Check sheet for the modelled part. Datum: model origin and axes. Units: mm. Round coordinates to 2 decimals unless told otherwise and drop trailing zeros. Order: outer loops, then holes, each group sorted by start corner. A loop starts at its lowest first (then second) coordinate and runs counter-clockwise, first axis right, second up. Notation, with made-up numbers: (-8, -1.5) -> (4, -1.5) arc R13 ccw to (4, 22.5) -> close; hole circle Ø8 at (-38.75, 19.5). An arc over 180 degrees is marked (long way). Answer in a Markdown table with one row per item. Add a question column.
1. Sectioned sample at D-D, the plane z = -24. Record the boundary of the cut face in (x, y), then the cut area to 3 significant figures.
2. Sectioned sample at B-B, the plane x = -32. Record the boundary of the cut face in (y, z).
3. Depth check by flat-ended pin: P1, Ø1.8, axis at x = 34.34, z = -80.5, coming from the +Y side. Enter the tip coordinate at first touch or a pass-through.
4. Sectioned sample at C-C, the plane x = 23. Record the boundary of the cut face in (y, z).
5. Sectioned sample at A-A, the plane z = -131. Record the boundary of the cut face in (x, y).
6. Material ranges on L1, parallel to X at y = 1.05, z = -55.5; L2, parallel to Z at x = -9.5, y = 0.45; L3, parallel to X at y = 1.65, z = -84, recorded low to high. Write a range as from..to.
Autodesk Inventor part; units mm, degrees
ref_plane "YZ Plane" through (0, 0, 0) normal (1, 0, 0) x (0, 1, 0)
ref_plane "XZ Plane" through (0, 0, 0) normal (0, 1, 0) x (-1, 0, 0)
ref_plane "XY Plane" through (0, 0, 0) normal (0, 0, 1) x (1, 0, 0)
sketch "Sketch1" plane through (0, 0, 0) normal (0, 1, 0) x (-1, 0, 0)
  line L0 (37.7589, 9.4959) -> (-42.2411, 9.4959)
  line L1 (-42.2411, 9.4959) -> (-42.2411, -290.5041)
  line L2 (-42.2411, -290.5041) -> (37.7589, -290.5041)
  line L3 (27.7589, -20.5041) -> (1.7589, -20.5041)
  line L4 (1.7589, -20.5041) -> (1.7589, -65.5041)
  line L5 (1.7589, -65.5041) -> (27.7589, -65.5041)
  line L6 (27.7589, -65.5041) -> (27.7589, -20.5041)
  line L7 (-8.2411, -20.5041) -> (-34.2411, -20.5041)
  line L8 (-34.2411, -20.5041) -> (-34.2411, -65.5041)
  line L9 (-34.2411, -65.5041) -> (-8.2411, -65.5041)
  line L10 (-8.2411, -65.5041) -> (-8.2411, -20.5041)
  line L11 (-6.2411, -81.8041) -> (-32.2411, -81.8041)
  line L12 (-32.2411, -81.8041) -> (-32.2411, -156.8041)
  line L13 (-32.2411, -156.8041) -> (-6.2411, -156.8041)
  line L14 (-6.2411, -156.8041) -> (-6.2411, -81.8041)
  circle A0 centre (-3.3411, -80.5041) radius 1.5
  circle A1 centre (-34.3411, -80.5041) radius 1.5
  circle A2 centre (-3.3411, -155.5041) radius 1.5
  circle A3 centre (-34.3411, -155.5041) radius 1.5
  line L15 (37.7589, 9.4959) -> (37.7589, -110.5041)
  line L16 (37.7589, -110.5041) -> (7.7589, -110.5041)
  line L17 (7.7589, -110.5041) -> (7.7589, -170.5041)
  line L18 (7.7589, -170.5041) -> (37.7589, -170.5041)
  line L19 (37.7589, -170.5041) -> (37.7589, -290.5041)
  line L20 (12.7589, -238.5041) -> (-17.2411, -238.5041)
  line L21 (-17.2411, -238.5041) -> (-17.2411, -260.5041)
  line L22 (-17.2411, -260.5041) -> (12.7589, -260.5041)
  line L23 (12.7589, -260.5041) -> (12.7589, -238.5041)
  line L24 (12.7589, -210.5041) -> (-6.2411, -210.5041)
  line L25 (-6.2411, -210.5041) -> (-6.2411, -223.5041)
  line L26 (-6.2411, -223.5041) -> (12.7589, -223.5041)
  line L27 (12.7589, -223.5041) -> (12.7589, -210.5041)
  circle A4 centre (-7.2411, -275.5041) radius 1.5
  circle A5 centre (-7.2411, -5.5041) radius 1.5
  point P0 (0, 0)
  dimension "d0" = 300
  dimension "d1" = 80
  dimension "d4" = 45
  dimension "d5" = 26
  dimension "d6" = 30
  dimension "d8" = 45
  dimension "d9" = 26
  dimension "d10" = 30
  dimension "d11" = 10
  dimension "d12" = 75
  dimension "d13" = 26
  dimension "d16" = 1.3
  dimension "d17" = 2.9
  dimension "d18" = 3
  dimension "d20" = 31
  dimension "d22" = 3
  dimension "d23" = 75
  dimension "d24" = 3
  dimension "d25" = 75
  dimension "d26" = 3
  dimension "d27" = 15
  dimension "d28" = 10
  dimension "d29" = 120
  dimension "d30" = 120
  dimension "d31" = 30
  dimension "d32" = 22
  dimension "d33" = 30
  dimension "d34" = 25
  dimension "d35" = 30
  dimension "d36" = 13
  dimension "d37" = 19
  dimension "d38" = 25
  dimension "d39" = 15
  dimension "d40" = 45
  dimension "d41" = 15
  dimension "d42" = 3
  dimension "d43" = 45
  dimension "d44" = 15
  dimension "d45" = 3
extrude "Extrusion1" add sketch "Sketch1" along normal blind 4
properties part number "support_arriere"
Answer key:
| question | item | result |
|---|---|---|
| 1 | outline | (-37.76, 0) -> (-27.76, 0) -> (-27.76, 4) -> (-37.76, 4) -> close; (-1.76, 0) -> (8.24, 0) -> (8.24, 4) -> (-1.76, 4) -> close; (34.24, 0) -> (42.24, 0) -> (42.24, 4) -> (34.24, 4) -> close |
| 1 | area | 112 mm² |
| 2 | outline | (0, -290.5) -> (4, -290.5) -> (4, -170.5) -> (0, -170.5) -> close; (0, -110.5) -> (4, -110.5) -> (4, 9.5) -> (0, 9.5) -> close |
| 3 | P1 | passes through |
| 4 | outline | (0, -290.5) -> (4, -290.5) -> (4, -156.8) -> (0, -156.8) -> close; (0, -81.8) -> (4, -81.8) -> (4, -65.5) -> (0, -65.5) -> close; (0, -20.5) -> (4, -20.5) -> (4, 9.5) -> (0, 9.5) -> close |
| 5 | outline | (-7.76, 0) -> (6.24, 0) -> (6.24, 4) -> (-7.76, 4) -> close; (32.24, 0) -> (42.24, 0) -> (42.24, 4) -> (32.24, 4) -> close |
| 6 | L1 | x = -37.76..-27.76, -1.76..8.24, 34.24..42.24 |
| 6 | L2 | z = -290.5..-260.5, -238.5..-223.5, -210.5..-170.5, -110.5..-65.5, -20.5..9.5 |
| 6 | L3 | x = -37.76..6.24, 32.24..42.24 |
